Can you work these out from the model? Positions are in its coordinate system, mm. A direction names the side the tool comes from. Coordinates: 2 decimals unless noted, no trailing zeros. Order: outer loops, then holes, each group sorted by start corner. A loop starts at its lowest first (then second) coordinate and runs counter-clockwise, first axis right, second up. Notation, with made-up numbers: (39.25, 41) -> (79.25, 41) arc R19 ccw to (79.25, 58) -> close; hole circle Ø6 at (74, -38.5). An arc over 180 degrees is marked (long way). Use a Markdown table: item, result. Add a question column.
1. For faces 5 (the cylindrical face through (-12.932, 5.362, 3.986)), 6 (the flat face through (0, 18, 1)), which set-ups out of +Z, -Z, +X, -X, +Y, -Y let a thin tool reach every point of the face, with its end or its side?
2. For pin 1 Ø4.5 at (x, y) = (14.14, 14.14) entering from -Z; pin 2 Ø2.5 at (x, y) = (-14.14, 14.14) entering from +Z, each with a flat end and sliding along its axis, tell me the tip position at first contact or that it passes through.
3. We'd pull the mould along X, two halves only. Please class faces 1 (the flat face through (-12.3, 4.3, 0)), 2 (the flat face through (18, 0, 1)), 3 (the cylindrical face through (14.93, -15.65, 2.34)), 4 (the cylindrical face through (-15.49, -15.18, 2.34)): pulls with the +X half, pulls with the -X half, needs draft (parallel to the pull), parting line crosses it, or undercut.
4. Suppose I cut it at D-D, the plane x = 15. State how many separate pieces and enclosed holes the cut face has, then the cut area to 3 significant figures.
5. Suppose I cut it at A-A, the plane y = 0. List the corners of the cut face in (x, z) for me.
6. If I drill on line 1 along X through (y, z) = (-15.5, 2.15); line 2 along Y through (x, z) = (0, 1.9); line 3 along Y through (x, z) = (13, 1.05), over which ranges is the centre line in solid material (lowest first)? Write a range as from..to.
7. Suppose I cut it at C-C, the plane z = 2.35. List the corners of the cut face in (x, y) for me.
```python
from build123d import *

# Parameters (mm, degrees)
ESBO_O1_W                            = 36
ESBO_O1_H                            = 36
ESBO_O1_R                            = 12.5
RESSALTO_EXTRUS_O1_DEPTH             = 3
ESBO_O2_R                            = 14
ESBO_O2_R_2                          = 12.5
RESSALTO_EXTRUS_O2_DEPTH             = 2
ESCAREADO_PARA_SFHCS_M32_D           = 3.4
ESCAREADO_PARA_SFHCS_M32_CSINK_D     = 6.72
ESCAREADO_PARA_SFHCS_M32_CSINK_ANGLE = 90


with BuildPart() as part:
    # Esboço1 → Ressalto-extrusão1 (new body)
    with BuildSketch(Plane.XY):
        Rectangle(ESBO_O1_W, ESBO_O1_H)
        Circle(ESBO_O1_R, mode=Mode.SUBTRACT)
    extrude(amount=RESSALTO_EXTRUS_O1_DEPTH)

    # Esboço2 → Ressalto-extrusão2 (add)
    with BuildSketch(Plane.XY.offset(3)):
        with Locations(Location((0, 0, 0), (0, 0, 180))):
            Circle(ESBO_O2_R)
        Circle(ESBO_O2_R_2, mode=Mode.SUBTRACT)
    extrude(amount=RESSALTO_EXTRUS_O2_DEPTH)

    # Escareado para SFHCS M32 (through all)
    with Locations(Plane(origin=(0, 0, 0), x_dir=(-1, 0, 0), z_dir=(0, 0, -1))):
        with Locations((-14.142135624, 14.142135624), (14.142135624, 14.142135624), (14.142135624, -14.142135624), (-14.142135624, -14.142135624)):
            CounterSinkHole(ESCAREADO_PARA_SFHCS_M32_D / 2, ESCAREADO_PARA_SFHCS_M32_CSINK_D / 2, counter_sink_angle=ESCAREADO_PARA_SFHCS_M32_CSINK_ANGLE)


solid = part.part
```
Worked out:
| question | item | result |
|---|---|---|
| 1 | face 5 | +Z |
| 1 | face 6 | +Z, -Z, +X, -X, +Y |
| 2 | pin 1 | stops at z = 1.11 |
| 2 | pin 2 | passes through |
| 3 | face 1 | needs draft |
| 3 | face 2 | pulls with the +X half |
| 3 | face 3 | undercut |
| 3 | face 4 | undercut |
| 4 | separate pieces | 3 |
| 4 | enclosed holes | 0 |
| 4 | area | 84.4 mm² |
| 5 | outline | (-18, 0) -> (-12.5, 0) -> (-12.5, 5) -> (-14, 5) -> (-14, 3) -> (-18, 3) -> close; (12.5, 0) -> (18, 0) -> (18, 3) -> (14, 3) -> (14, 5) -> (12.5, 5) -> close |
| 6 | line 1 | x = -18..-15.16, -13.12..13.12, 15.16..18 |
| 6 | line 2 | y = -18..-12.5, 12.5..18 |
| 6 | line 3 | y = -18..-16.15, -12.13..12.13, 16.15..18 |
| 7 | outline | (-18, -18) -> (18, -18) -> (18, 18) -> (-18, 18) -> close; hole circle Ø3.4 at (-14.14, -14.14); hole circle Ø3.4 at (-14.14, 14.14); hole circle Ø25 at (0, 0); hole circle Ø3.4 at (14.14, -14.14); hole circle Ø3.4 at (14.14, 14.14) |
